Check sheet for the modelled part. Datum: model origin and axes. Units: mm. Face numbers are marked on the shaded views. A direction names the side the tool comes from. Round coordinates to 2 decimals unless told otherwise and drop trailing zeros. Write each loop counter-clockwise with the first axis right and the second up, starting at its lowest first coordinate (ties: lowest second). Pieces come first, ordered by that corner, then holes.
Item 1: Release check for a two-part mould opening along X. For the marked faces 1, 2 and 3 record: pulls with the +X half, pulls with the -X half, needs draft (parallel to the pull), parting line crosses it, or undercut.
Item 2: Section check D-D, the plane y = 3. Record the cut outline in (x, z) (3 decimals).
Item 3: Depth check by flat-ended pin: pin 1 (12 mm diameter, centred on x = -9.5, z = -14.5, fed in from +Y); pin 2 (4.5 mm diameter, centred on x = 21.5, y = 5, fed in from -Z); pin 3 (2.5 mm diameter, centred on y = 11.5, z = -24.5, fed in from -X); pin 4 (3 mm diameter, centred on x = -22.5, z = 0, fed in from -Y). Enter the tip coordinate at first touch or a pass-through.
Item 4: Section check B-B, the plane x = 0. Record the cut outline in (y, z).
Item 5: Section check A-A, the plane y = 10.75. Record the cut outline in (x, z) (3 decimals).
Item 6: Material ranges on line 1 along Z through (x, y) = (11.5, 5.5); line 2 along Z through (x, y) = (24, 7.5); line 3 along Y through (x, z) = (9, 9), recorded low to high.
Item 7: Section check C-C, the plane z = 3.5. Record the cut outline in (x, y) (3 decimals), plus the area to 3 significant figures.
Item 8: Set-up check for the marked faces 4, 5 and 6: record each of +Z, -Z, +X, -X, +Y, -Y from which the full face is reachable in a straight line by a thin tool's end or side.
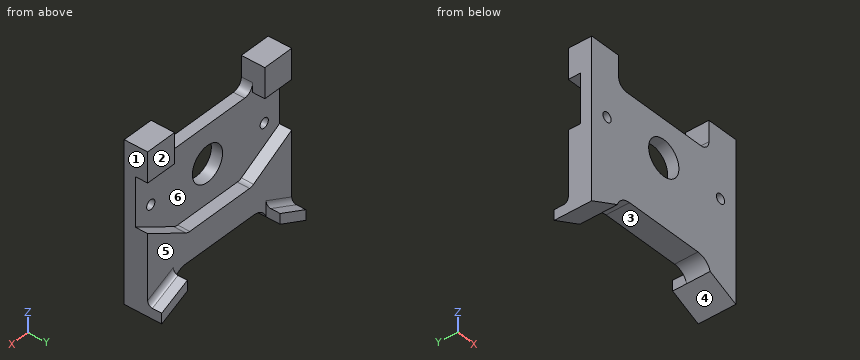
from build123d import *

# Parameters (mm, degrees)
SKETCH1_W             = 57.15
SKETCH1_H             = 25.4
BOSS_EXTRUDE1_DEPTH   = 3.81
CUT_EXTRUDE1_REACH    = 33.501
SKETCH2_R             = 6
F_4_CLEARANCE_HOLE1_D = 3.2639
BOSS_EXTRUDE4_DEPTH   = 3.81
BOSS_EXTRUDE5_DEPTH   = 8.89
SKETCH12_W            = 36.83
SKETCH12_H            = 9.899955096
BOSS_EXTRUDE6_DEPTH   = 3.81
BOSS_EXTRUDE7_DEPTH   = 4.1275
FILLET4_R             = 3.175
FILLET5_R             = 1.5875
BOSS_EXTRUDE8_REACH   = 45.92
SKETCH14_W            = 10.668
SKETCH14_H            = 10.16
FILLET6_R             = 3.175
FILLET7_R             = 5.08


with BuildPart() as part:
    # Sketch1 → Boss-Extrude1 (new body)
    with BuildSketch(Plane(origin=(0, 0, 0), x_dir=(1, 0, 0), z_dir=(0, 1, 0))):
        Rectangle(SKETCH1_W, SKETCH1_H)
    extrude(amount=BOSS_EXTRUDE1_DEPTH)

    # Sketch2 → Cut-Extrude1 (cut, up to next)
    with BuildSketch(Plane(origin=(0, 3.81, 0), x_dir=(1, 0, 0), z_dir=(0, 1, 0)), mode=Mode.PRIVATE) as cut_extrude1_sk1:
        with Locations(Location((0, 0, 0), (0, 0, 270))):
            Circle(SKETCH2_R)
    cut_extrude1_tool1 = extrude(cut_extrude1_sk1.sketch, amount=-CUT_EXTRUDE1_REACH, mode=Mode.PRIVATE) & part.part
    add(cut_extrude1_tool1.solids().sort_by_distance((0, 3.81, 0))[0], mode=Mode.SUBTRACT)

    # #4 Clearance Hole1 (through all)
    with Locations(Plane(origin=(0, 3.81, 0), x_dir=(1, 0, 0), z_dir=(0, 1, 0))):
        with Locations((-22.5, 0), (22.5, 0)):
            Hole(F_4_CLEARANCE_HOLE1_D / 2)

    # Sketch8 → Boss-Extrude4 (add)
    with BuildSketch(Plane(origin=(0, 3.81, 0), x_dir=(1, 0, 0), z_dir=(0, 1, 0))):
        Polygon((-28.575, 30.840865795), (-28.575, 12.7), (-18.415, 12.7), (-18.415, 26.103179988), align=None)
    boss_extrude4 = extrude(amount=-BOSS_EXTRUDE4_DEPTH)

    # Mirror4: Boss-Extrude4 across plane
    add(boss_extrude4.mirror(Plane(origin=(0, 0, 0), x_dir=(0, 0, 1), z_dir=(1, 0, 0))))

    # Sketch11 → Boss-Extrude5 (add)
    with BuildSketch(Plane(origin=(0, 3.81, 0), x_dir=(1, 0, 0), z_dir=(0, 1, 0))):
        Polygon((-18.415, 26.103179988), (-28.575, 30.840865795), (-28.575, 27.337640903), (-18.415, 22.599955096), align=None)
    boss_extrude5 = extrude(amount=BOSS_EXTRUDE5_DEPTH)

    # Mirror7: Boss-Extrude5 across plane
    add(boss_extrude5.mirror(Plane(origin=(0, 0, 0), x_dir=(0, 0, 1), z_dir=(1, 0, 0))))

    # Sketch12 → Boss-Extrude6 (add)
    with BuildSketch(Plane(origin=(0, 3.81, 0), x_dir=(1, 0, 0), z_dir=(0, 1, 0))):
        with Locations((0, 17.649977548)):
            Rectangle(SKETCH12_W, SKETCH12_H)
    extrude(amount=-BOSS_EXTRUDE6_DEPTH)

    # Sketch13 → Boss-Extrude7 (add)
    with BuildSketch(Plane(origin=(0, 3.81, 0), x_dir=(1, 0, 0), z_dir=(0, 1, 0))):
        Polygon((12.7, 12.947955096), (-12.7, 12.947955096), (-28.575, 3.782519572), (-28.575, 27.337640903), (-18.415, 22.599955096), (18.415, 22.599955096), (28.575, 27.337640903), (28.575, 3.782519572), align=None)
    extrude(amount=BOSS_EXTRUDE7_DEPTH)

    # Fillet4
    fillet4_edges = [part.edges().sort_by_distance(p)[0] for p in [
        (-12.7, 5.87375, -12.947955096),
        (12.7, 5.87375, -12.947955096),
    ]]
    fillet(fillet4_edges, radius=FILLET4_R)

    # Fillet5
    fillet5_edges = [part.edges().sort_by_distance(p)[0] for p in [
        (23.495, 7.9375, -24.968797999),
        (-23.495, 7.9375, -24.968797999),
    ]]
    fillet(fillet5_edges, radius=FILLET5_R)

    # Boss-Extrude8: up to this face of the body (flat: up to its plane)
    boss_extrude8_end = Plane(part.part.faces().sort_by_distance((0, 7.9375, -16.275006061))[0])
    # Sketch14 → Boss-Extrude8 (add, up to the picked face)
    with BuildSketch(Plane(origin=(0, 0, 0), x_dir=(1, 0, 0), z_dir=(0, 1, 0)), mode=Mode.PRIVATE) as boss_extrude8_sk1:
        with Locations((23.241, -17.78)):
            Rectangle(SKETCH14_W, SKETCH14_H)
    boss_extrude8_tool1 = split(extrude(boss_extrude8_sk1.sketch, amount=BOSS_EXTRUDE8_REACH, mode=Mode.PRIVATE), bisect_by=boss_extrude8_end, keep=Keep.BOTH, mode=Mode.PRIVATE)
    boss_extrude8 = boss_extrude8_tool1.solids().sort_by(Axis((23.241, 0, 17.78), (0, 1, 0)))[0]
    add(boss_extrude8)

    # Mirror9: Boss-Extrude8 across plane
    add(boss_extrude8.mirror(Plane(origin=(0, 0, 0), x_dir=(0, 0, 1), z_dir=(1, 0, 0))))

    # Fillet6
    fillet6_edges = [part.edges().sort_by_distance(p)[0] for p in [
        (17.907, 1.905, 12.7),
        (-17.907, 1.905, 12.7),
    ]]
    fillet(fillet6_edges, radius=FILLET6_R)

    # Fillet7
    # the kernel refuses this fillet: 5.08 mm, written as the material it adds along each edge
    with BuildSketch(Plane(origin=(-18.415, 0, -22.599955096), x_dir=(0, 0, -1), z_dir=(0, 1, 0))) as fillet7_piece_1:
        with BuildLine():
            CenterArc((5.08, -4.829097251), FILLET7_R, 108.082662978, 71.917337022)
            Line((0, -4.829097251), (-0.1016, -4.829097251))
            Line((-0.1016, -4.829097251), (-0.1016, 0))
            Line((-0.1016, 0), (0, 0.1016))
            ThreePointArc((0, 0.1016), (1.751612446, 0.1016), (3.471689391, 0.096581945))
            Line((3.471689391, 0.096581945), (3.503224893, 0))
        make_face()
    extrude(amount=7.9375)
    with BuildSketch(Plane(origin=(18.415, 0, -22.599955096), x_dir=(0, 0, -1), z_dir=(0, 1, 0))) as fillet7_piece_2:
        with BuildLine():
            CenterArc((5.08, 4.829097251), FILLET7_R, 180, 71.917337022)
            Line((0, 4.829097251), (-0.1016, 4.829097251))
            Line((-0.1016, 4.829097251), (-0.1016, 0))
            Line((-0.1016, 0), (0, -0.1016))
            ThreePointArc((0, -0.1016), (1.751612446, -0.1016), (3.471689391, -0.096581945))
            Line((3.471689391, -0.096581945), (3.503224893, 0))
        make_face()
    extrude(amount=7.9375)


solid = part.part
Values found:
1. face 1: pulls with the +X half
1. face 2: needs draft
1. face 3: undercut
2. outline: (-28.575, -30.841) - (-18.415, -26.103) arc R5.08 cw to (-13.586, -22.6) - (13.586, -22.6) arc R5.08 cw to (18.415, -26.103) - (28.575, -30.841) - (28.575, 22.86) - (17.907, 22.86) - (17.907, 15.875) arc R3.175 cw to (14.732, 12.7) - (-14.732, 12.7) arc R3.175 cw to (-17.907, 15.875) - (-17.907, 22.86) - (-28.575, 22.86) - close; hole circle Ø3.264 at (-22.5, 0); hole circle Ø12 at (0, 0); hole circle Ø3.264 at (22.5, 0)
3. pin 1: stops at y = 7.94
3. pin 2: stops at z = -28.59
3. pin 3: stops at x = -25.17
3. pin 4: passes through
4. outline: (0, -22.6) - (7.94, -22.6) - (7.94, -12.95) - (3.81, -12.95) - (3.81, -6) - (0, -6) - close; (0, 6) - (3.81, 6) - (3.81, 12.7) - (0, 12.7) - close
5. outline: (-28.575, -30.841) - (-18.415, -26.103) - (-18.415, -22.6) - (-28.575, -27.338) - close; (18.415, -26.103) - (28.575, -30.841) - (28.575, -27.338) - (18.415, -22.6) - close
6. line 1: z = -22.6 to -12.95
6. line 2: z = -28.71 to -6.42, 12.7 to 22.86
6. line 3: y = 0 to 3.81
7. outline: (-28.575, 0) - (-4.873, 0) - (-4.873, 3.81) - (-28.575, 3.81) - close; (4.873, 0) - (28.575, 0) - (28.575, 3.81) - (4.873, 3.81) - close
7. area: 181 mm2
8. face 4: -Z, +Y, -Y
8. face 5: +Z, +Y
8. face 6: +Y
